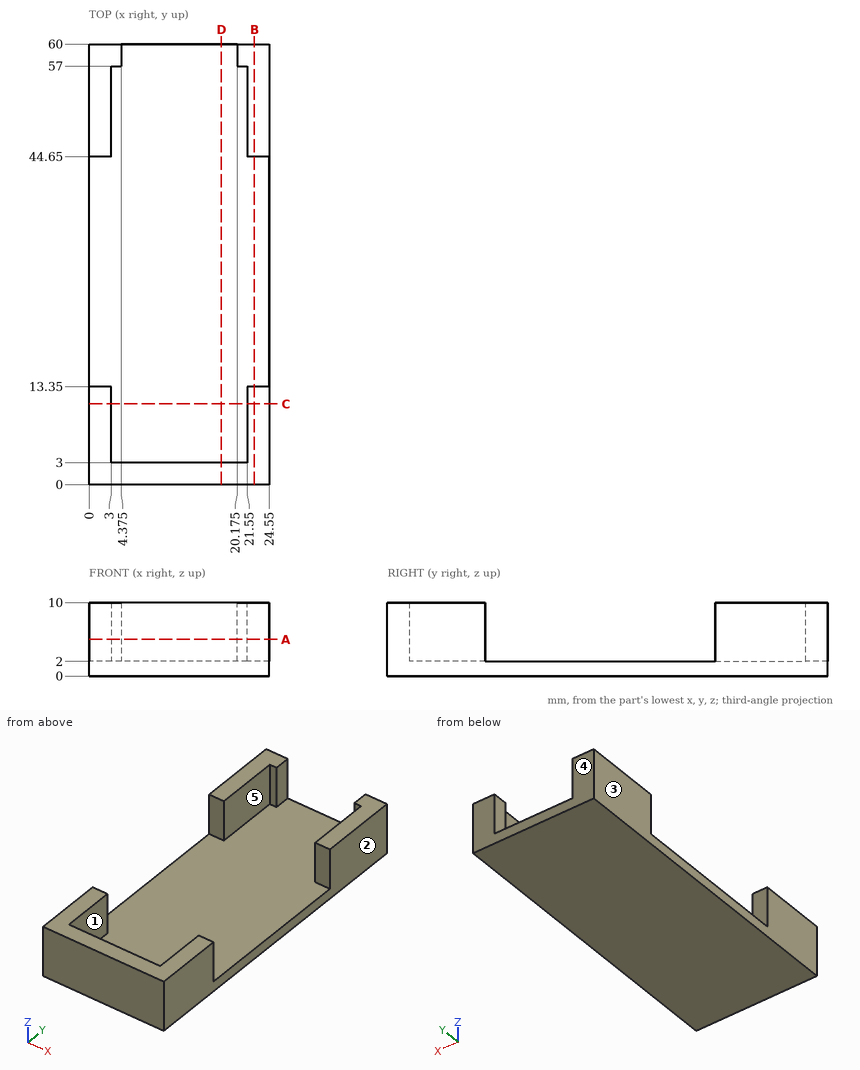
Verification items for this drawing (mm, ordinates from the low corner). A direction names the side the tool comes from. Round coordinates to 2 decimals unless told otherwise and drop trailing zeros. Order: outer loops, then holes, each group sorted by start corner. A loop starts at its lowest first (then second) coordinate and runs counter-clockwise, first axis right, second up. Notation, with made-up numbers: (44.25, 34) -> (73.25, 34) arc R18 cw to (73.25, 54) -> close; hole circle Ø9 at (-30, 76.25). An arc over 180 degrees is marked (long way). Use one line per item in the form item = value.
1. Cross-section at D-D, the plane x = 18. Enter the section's corners in (y, z).
Working result:
outline = (0, 0) -> (60, 0) -> (60, 2) -> (3, 2) -> (3, 10) -> (0, 10) -> close
2. Cross-section at A-A, the plane z = 5. Enter the section's corners in (x, y) (3 decimals).
Working result:
outline = (0, 0) -> (24.55, 0) -> (24.55, 13.35) -> (21.55, 13.35) -> (21.55, 3) -> (3, 3) -> (3, 13.35) -> (0, 13.35) -> close; (0, 44.65) -> (3, 44.65) -> (3, 57) -> (4.375, 57) -> (4.375, 60) -> (0, 60) -> close; (20.175, 57) -> (21.55, 57) -> (21.55, 44.65) -> (24.55, 44.65) -> (24.55, 60) -> (20.175, 60) -> close
3. Go/stop test with a flat-tipped pin: pin 1 (12.5 mm diameter, centred on x = 7, y = 33, fed in from +Z). Record where the tip stops, or that it passes through.
Working result:
pin_1 = 2
4. Cross-section at B-B, the plane x = 22.5. Enter the section's corners in (y, z), plus the area to 3 significant figures.
Working result:
outline = (0, 0) -> (60, 0) -> (60, 10) -> (44.65, 10) -> (44.65, 2) -> (13.35, 2) -> (13.35, 10) -> (0, 10) -> close
area = 350 mm^2
5. Scan lines: line 1 along X through (y, z) = (9, 9.5); line 2 along Y through (x, z) = (22.5, 9); line 3 along Y through (x, z) = (20.5, 9.5). Record each from-to range of solid material in increasing order. Write a range as from..to.
Working result:
line_1 = 0..3, 21.55..24.55
line_2 = 0..13.35, 44.65..60
line_3 = 0..3, 57..60
6. Mould release check, pull along X, two halves, no side actions. Record for the marked faces 1, 2 and 3: pulls with the +X half, pulls with the -X half, needs draft (parallel to the pull), parting line crosses it, or undercut.
Working result:
face_1 = undercut
face_2 = pulls with the +X half
face_3 = pulls with the -X half
7. Cross-section at C-C, the plane y = 11. Enter the section's corners in (x, z).
Working result:
outline = (0, 0) -> (24.55, 0) -> (24.55, 10) -> (21.55, 10) -> (21.55, 2) -> (3, 2) -> (3, 10) -> (0, 10) -> close
8. Set-up check for the marked faces 4 and 5: record each of +Z, -Z, +X, -X, +Y, -Y from which the full face is reachable in a straight line by a thin tool's end or side.
Working result:
face_4 = +Z, -Z, +X, -X, +Y
face_5 = +Z
